from build123d import *

# Parameters (mm, degrees)
EXTRUDE068_DEPTH           = 3
EXTRUDE068_PLACEMENT_ANGLE = 180
EXTRUDE067_DEPTH           = 3
EXTRUDE027_DEPTH           = 3.5
EXTRUDE034_DEPTH           = 3.5
EXTRUDE034_PLACEMENT_ANGLE = 180
EXTRUDE020_DEPTH           = 2.5
EXTRUDE019_DEPTH           = 6.25
CUT036_PLACEMENT_ANGLE     = 90


with BuildPart() as extrude068:
    # Sketch040 → Extrude068 (new body)
    with BuildSketch(Plane.XZ):
        with BuildLine():
            Line((32.579475, 2.855954), (34.598949, 2.855954))
            Line((34.598949, 2.855954), (34.598949, -1.799177))
            Line((34.598949, -1.799177), (33.872559, -1.799177))
            Line((33.872559, -1.799177), (31.075473, -0.756428))
            ThreePointArc((31.172102, -0.672237), (31.109316, -0.697722), (31.075473, -0.756428))
            Line((32.386694, -0.781542), (31.172102, -0.672237))
            ThreePointArc((32.386694, -0.781542), (33.712242, -0.224592), (34.260406, 1.104614))
            ThreePointArc((34.260406, 1.104614), (33.763902, 2.113863), (32.714019, 2.517408))
            ThreePointArc((32.579475, 2.855954), (32.532862, 2.641421), (32.714019, 2.517408))
        make_face()
    extrude(amount=EXTRUDE068_DEPTH)


with BuildPart() as extrude068_1:
    # Extrude068 placement: moved
    add(extrude068.part.moved(Location((84.4, -62.8, 0))).rotate(Axis((84.4, -62.8, 0), (0, 0, 1)), EXTRUDE068_PLACEMENT_ANGLE))


with BuildPart() as extrude067:
    # Sketch040 → Extrude067 (new body)
    with BuildSketch(Plane.XZ):
        with BuildLine():
            Line((32.579475, 2.855954), (34.598949, 2.855954))
            Line((34.598949, 2.855954), (34.598949, -1.799177))
            Line((34.598949, -1.799177), (33.872559, -1.799177))
            Line((33.872559, -1.799177), (31.075473, -0.756428))
            ThreePointArc((31.172102, -0.672237), (31.109316, -0.697722), (31.075473, -0.756428))
            Line((32.386694, -0.781542), (31.172102, -0.672237))
            ThreePointArc((32.386694, -0.781542), (33.712242, -0.224592), (34.260406, 1.104614))
            ThreePointArc((34.260406, 1.104614), (33.763902, 2.113863), (32.714019, 2.517408))
            ThreePointArc((32.579475, 2.855954), (32.532862, 2.641421), (32.714019, 2.517408))
        make_face()
    extrude(amount=EXTRUDE067_DEPTH)


with BuildPart() as extrude067_1:
    # Extrude067 placement: moved
    add(extrude067.part.moved(Location((0, -59.8, 0))))


with BuildPart() as extrude027:
    # Sketch019 → Extrude027 (new body)
    with BuildSketch(Plane.XZ):
        with BuildLine():
            Line((82.710403, -2.436997), (80.667656, -0.042506))
            Line((80.667656, -0.042506), (62.164684, -0.042506))
            Line((62.164684, -0.042506), (58.594872, -2.493932))
            Line((58.594872, -2.493932), (64.198559, -2.493932))
            Line((64.198559, -2.493932), (64.198559, -6.97036))
            Line((64.198559, -6.97036), (65.852661, -6.97036))
            Line((65.852661, -6.97036), (65.852661, -1.924586))
            ThreePointArc((66.964828, -0.767347), (66.162314, -1.109134), (65.852661, -1.924586))
            Line((66.964828, -0.767347), (73.098848, -0.767347))
            ThreePointArc((74.177399, -1.907358), (73.865032, -1.122677), (73.098848, -0.767347))
            Line((74.177399, -1.907358), (74.177399, -7.098253))
            Line((74.177399, -7.098253), (75.826362, -7.098253))
            Line((75.826362, -7.098253), (75.826362, -2.436997))
            Line((75.826362, -2.436997), (82.710403, -2.436997))
        make_face()
    extrude(amount=EXTRUDE027_DEPTH)


with BuildPart() as extrude027_1:
    # Extrude027 placement: moved
    add(extrude027.part.moved(Location((0.12, -61, 0))))


with BuildPart() as extrude034:
    # Sketch019 → Extrude034 (new body)
    with BuildSketch(Plane.XZ):
        with BuildLine():
            Line((82.710403, -2.436997), (80.667656, -0.042506))
            Line((80.667656, -0.042506), (62.164684, -0.042506))
            Line((62.164684, -0.042506), (58.594872, -2.493932))
            Line((58.594872, -2.493932), (64.198559, -2.493932))
            Line((64.198559, -2.493932), (64.198559, -6.97036))
            Line((64.198559, -6.97036), (65.852661, -6.97036))
            Line((65.852661, -6.97036), (65.852661, -1.924586))
            ThreePointArc((66.964828, -0.767347), (66.162314, -1.109134), (65.852661, -1.924586))
            Line((66.964828, -0.767347), (73.098848, -0.767347))
            ThreePointArc((74.177399, -1.907358), (73.865032, -1.122677), (73.098848, -0.767347))
            Line((74.177399, -1.907358), (74.177399, -7.098253))
            Line((74.177399, -7.098253), (75.826362, -7.098253))
            Line((75.826362, -7.098253), (75.826362, -2.436997))
            Line((75.826362, -2.436997), (82.710403, -2.436997))
        make_face()
    extrude(amount=EXTRUDE034_DEPTH)


with BuildPart() as extrude034_1:
    # Extrude034 placement: moved
    add(extrude034.part.moved(Location((83.88, -64.6, 0))).rotate(Axis((83.88, -64.6, 0), (0, 0, 1)), EXTRUDE034_PLACEMENT_ANGLE))


with BuildPart() as extrude020:
    # Sketch012 → Extrude020 (new body)
    with BuildSketch(Plane.XY):
        with BuildLine():
            ThreePointArc((22.35, 0.5), (42.5, -6.665278), (62.65, 0.5))
            Line((59.35, 5.5), (62.65, 0.5))
            Line((25.6, 5.5), (59.35, 5.5))
            Line((22.35, 0.5), (25.6, 5.5))
        make_face()
        with BuildLine():
            Line((26.5, 3.25), (58.5, 3.25))
            ThreePointArc((59, 0.854356), (59.723633, 2.255387), (58.5, 3.25))
            Line((59, 0.854356), (50.5, -2.395644))
            Line((50.5, -2.395644), (34.5, -2.395644))
            Line((34.5, -2.395644), (26, 0.854356))
            ThreePointArc((26.5, 3.25), (25.276367, 2.255387), (26, 0.854356))
        make_face(mode=Mode.SUBTRACT)
        Polygon((21.85, 0.5), (0.5, 0.5), (0.5, 2.5), (19, 5.5), (25.06863, 5.5), align=None)
        Polygon((63.15, 0.5), (59.897327, 5.5), (66, 5.5), (84.5, 2.5), (84.5, 0.5), align=None)
    extrude(amount=EXTRUDE020_DEPTH)


with BuildPart() as extrude020_1:
    # Extrude020 placement: moved
    add(extrude020.part.moved(Location((0, 0, 3.75))))


with BuildPart() as seitentraeger:
    # Sketch011 → Extrude019 (new body)
    with BuildSketch(Plane.XY):
        with BuildLine():
            Line((22, 0), (0, 0))
            Line((0, 0), (0, 3))
            Line((0, 3), (19, 6))
            Line((19, 6), (66, 6))
            Line((66, 6), (85, 3))
            Line((85, 3), (85, 0))
            Line((85, 0), (63, 0))
            ThreePointArc((22, 0), (42.5, -7.28096), (63, 0))
        make_face()
        with BuildLine():
            Line((26.5, 2.85), (58.5, 2.85))
            ThreePointArc((58.857785, 1.228968), (59.330023, 2.183198), (58.5, 2.85))
            Line((58.857785, 1.228968), (50.661382, -1.8))
            Line((50.661382, -1.8), (34.364024, -1.8))
            Line((34.364024, -1.8), (26.164024, 1.219218))
            ThreePointArc((26.5, 2.85), (25.667484, 2.171516), (26.164024, 1.219218))
        make_face(mode=Mode.SUBTRACT)
    extrude(amount=EXTRUDE019_DEPTH)

    # Cut036: cut Extrude020
    add(extrude020_1.part, mode=Mode.SUBTRACT)


with BuildPart() as seitentraeger_1:
    # Cut036 placement: moved
    add(seitentraeger.part.moved(Location((-0.5, -59.8, 0))).rotate(Axis((-0.5, -59.8, 0), (1, 0, 0)), CUT036_PLACEMENT_ANGLE))

    # Fusion034: union Extrude027, Extrude034
    add(extrude027_1.part)
    add(extrude034_1.part)

    # Fusion058: union Extrude068, Extrude067
    add(extrude068_1.part)
    add(extrude067_1.part)


solid = seitentraeger_1.part
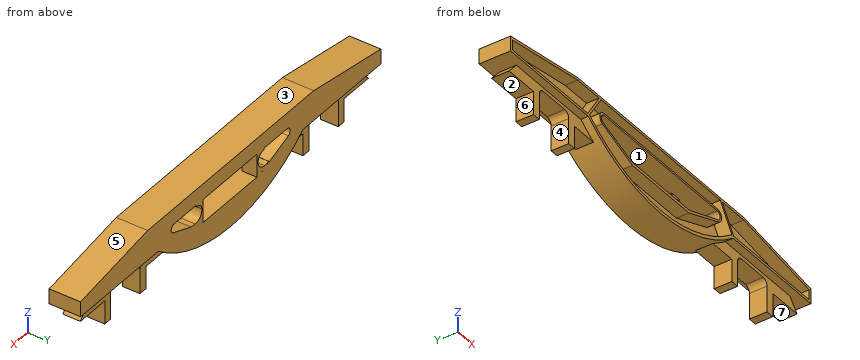
Geometry: final body of the model. Coordinates: model frame, mm. Face numbers are marked on the shaded views. A direction names the side the tool comes from. Give positions to 0.01 mm unless a question says otherwise; leave off trailing zeros. Write each loop counter-clockwise with the first axis right and the second up, starting at its lowest first coordinate (ties: lowest second). Pieces come first, ordered by that corner, then holes.
(1) Cut plane A-A, the plane x = 38. Return loops of the section in (y, z), then the cut area to 3 significant figures.
(2) First-contact query: P1, Ø3, axis at x = 72, y = -62.5, coming from the +Z side; P2, Ø1, axis at y = -62, z = -5.5, coming from the -X side; P3, Ø1.2, axis at x = 35, y = -64.5, coming from the -Z side. Flat tips, straight axial feed; report the tip coordinate or a pass-through.
(3) Access query for the marked faces 4, 5, 6 and 7. Directions: +Z, -Z, +X, -X, +Y, -Y. A direction counts if a zero-diameter tool reaches every point of the face in a straight line with its end or side. Return the directions, or none.
(4) Ray query, line 1 (Z direction, x = 30.5, y = -65.5); line 2 (Y direction, x = 62, z = 2); line 3 (Z direction, x = 19.5, y = -60.5). Return the intervals inside material, ascending.
(5) Mould query, pull axis Z, two halves, no side actions, for the marked faces 1, 2 and 3. Classes: released by +Z, released by -Z, zero draft, split by the parting line, or undercut.
(6) Cut plane D-D, the plane x = 14. Return loops of the section in (y, z).
(7) Cut plane B-B, the plane x = 60.5. Return loops of the section in (y, z), then the cut area to 3 significant figures.
Values follow:
1. outline: (-66.05, -7.03) - (-59.8, -7.03) - (-59.8, -1.8) - (-66.05, -1.8) - (-66.05, -2.4) - (-63.55, -2.4) - (-63.55, -6.41) - (-66.05, -6.41) - close; (-66.05, 2.85) - (-59.8, 2.85) - (-59.8, 6) - (-66.05, 6) - (-66.05, 5.5) - (-63.55, 5.5) - (-63.55, 3.25) - (-66.05, 3.25) - close
1. area: 36.7 mm2
2. P1: stops at z = 5.21
2. P2: stops at x = 8.05
2. P3: stops at z = -6.64
3. face 4: -Z, +Y, -Y
3. face 5: +Z, +X, +Y, -Y
3. face 6: -Z, -X, +Y, -Y
3. face 7: -Z, +X, +Y, -Y
4. line 1: z = -5.18 to -4.52, -1.06 to -0.56, 2.85 to 3.25, 5.5 to 6
4. line 2: y = -63.55 to -59.8
4. line 3: z = 0 to 6
5. face 1: undercut
5. face 2: released by -Z
5. face 3: released by +Z
6. outline: (-66.05, 0) - (-59.8, 0) - (-59.8, 5.29) - (-66.05, 5.29) - (-66.05, 4.77) - (-63.55, 4.77) - (-63.55, 0.5) - (-66.05, 0.5) - close; (-64.6, -0.77) - (-61.1, -0.77) - (-61.1, -0.04) - (-64.6, -0.04) - close
7. outline: (-66.05, -1.5) - (-64.5, -1.5) - (-64.5, -2.49) - (-61, -2.49) - (-61, -1.5) - (-59.8, -1.5) - (-59.8, 6) - (-66.05, 6) - (-66.05, 5.5) - (-63.55, 5.5) - (-63.55, 3.8) - (-66.05, 3.8) - (-66.05, 3) - (-63.55, 3) - (-63.55, -0.76) - (-66.05, -0.76) - close
7. area: 36.7 mm2
